Here's how the part is built. I have some questions about the finished solid (model axes, mm). Round coordinates to 2 decimals unless told otherwise and drop trailing zeros. Order: outer loops, then holes, each group sorted by start corner. A loop starts at its lowest first (then second) coordinate and runs counter-clockwise, first axis right, second up.
```python
from build123d import *

# Parameters (mm, degrees)
SKETCH1_W              = 25.4
SKETCH1_H              = 50.8
SKETCH1_W_2            = 22.225
SKETCH1_H_2            = 47.625
BOSS_EXTRUDE1_DEPTH    = 330.2
F_10_CLEARANCE_HOLE1_D = 5.1054


with BuildPart() as part:
    # Sketch1 → Boss-Extrude1 (new, symmetric)
    with BuildSketch(Plane(origin=(0, 0, 0), x_dir=(0, 0, -1), z_dir=(1, 0, 0))):
        with Locations((1.923003206, 0)):
            Rectangle(SKETCH1_W, SKETCH1_H)
        with Locations((1.923003206, 0)):
            Rectangle(SKETCH1_W_2, SKETCH1_H_2, mode=Mode.SUBTRACT)
    extrude(amount=BOSS_EXTRUDE1_DEPTH, both=True)

    # #10 Clearance Hole1 (through all)
    with Locations(Plane(origin=(0, 0, -14.623003206), x_dir=(-1, 0, 0), z_dir=(0, 0, -1))):
        with Locations((-241.3, 12.7), (-222.832275442, -4.738553542)):
            Hole(F_10_CLEARANCE_HOLE1_D / 2)


solid = part.part
```
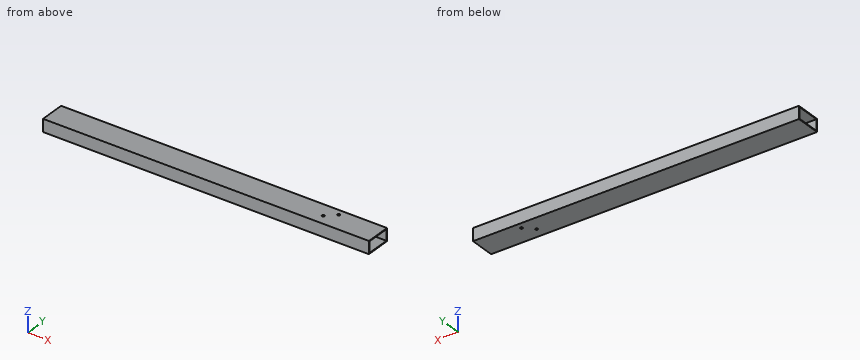
1. If we section it at B-B, the plane y = -14.5: Write out the boundary of the cut face in (x, z), and give its area (3 significant figures).
Evaluation:
outline: (-330.2, -14.62) - (330.2, -14.62) - (330.2, -13.04) - (-330.2, -13.04) - close; (-330.2, 9.19) - (330.2, 9.19) - (330.2, 10.78) - (-330.2, 10.78) - close
area: 2,100 mm2
2. I need wall thicknesses on probe 1 along Z at (x, y) = (244, 7); probe 2 along Y at (x, z) = (-116, -2); probe 3 along Y at (x, z) = (241.3, 9.8). Which ranges of each line are inside material? Lowest first, please.
Evaluation:
probe 1: z = -14.62 to -13.04, 9.19 to 10.78
probe 2: y = -25.4 to -23.81, 23.81 to 25.4
probe 3: y = -25.4 to 10.15, 15.25 to 25.4
3. If we section it at A-A, the plane z = -4: Write out the boundary of the cut face in (x, y).
Evaluation:
outline: (-330.2, -25.4) - (330.2, -25.4) - (330.2, -23.81) - (-330.2, -23.81) - close; (-330.2, 23.81) - (330.2, 23.81) - (330.2, 25.4) - (-330.2, 25.4) - close
4. If we section it at C-C, the plane x = 101: Write out the boundary of the cut face in (y, z).
Evaluation:
outline: (-25.4, -14.62) - (25.4, -14.62) - (25.4, 10.78) - (-25.4, 10.78) - close; hole (-23.81, -13.04) - (23.81, -13.04) - (23.81, 9.19) - (-23.81, 9.19) - close
5. I'm going to push a flat-ended pin straight in: P1, Ø6, axis at x = 222.83, y = -4.74, coming from the +Z side. Where does the tip first touch, or does it pass through?
Evaluation:
P1: stops at z = 10.78
